Here's the drawing with two shaded views (mm, measured from the low corner). I have some questions. A direction names the side the tool comes from. Give positions to 0.01 mm unless a question says otherwise; leave off trailing zeros. Loops run counter-clockwise (first coordinate to the right, second up) from the corner with the lowest first, then second, coordinate; pieces in that order, holes last. Notation, with made-up numbers: (36, -30) -> (56, -30) arc R21 ccw to (56, -21) -> close; hole circle Ø5 at (49.5, -31.75). An arc over 180 degrees is marked (long way). Answer in a Markdown table with one row per item. Add a question column.
Item 1: If we section it at D-D (x = 2.5): Write out the boundary of the cut face in (y, z).
Item 2: If we section it at B-B (z = 6.25): Write out the boundary of the cut face in (x, y).
Item 3: If I drill on line 1 (X direction, y = 5.5, z = 6.25); line 2 (Y direction, x = 5.5, z = 1); line 3 (X direction, y = 6.5, z = 4.5), over which ranges is the centre line in solid material (lowest first)?
Item 4: For P1, Ø3, axis at x = 6.5, y = 5, coming from the +Z side; P2, Ø4, axis at y = 4.5, z = 8.5, coming from the -X side; P3, Ø6, axis at y = 6.5, z = 11, coming from the +X side, each with a flat end and sliding along its axis, tell me the tip position at first contact or that it passes through.
Item 5: We'd pull the mould along X, two halves only. Please class the marked faces 1, 2 and 3: released by +X, released by -X, zero draft, split by the parting line, or undercut.
Item 6: If we section it at A-A (x = 6.25): Write out the boundary of the cut face in (y, z).
Item 7: Which directions (+Z, -Z, +X, -X, +Y, -Y) give clear straight access to the entire face, cutting with the end or side of a thin tool? Please do the marked faces 4 and 5.
Item 8: If we section it at C-C (y = 4): Write out the boundary of the cut face in (x, z).
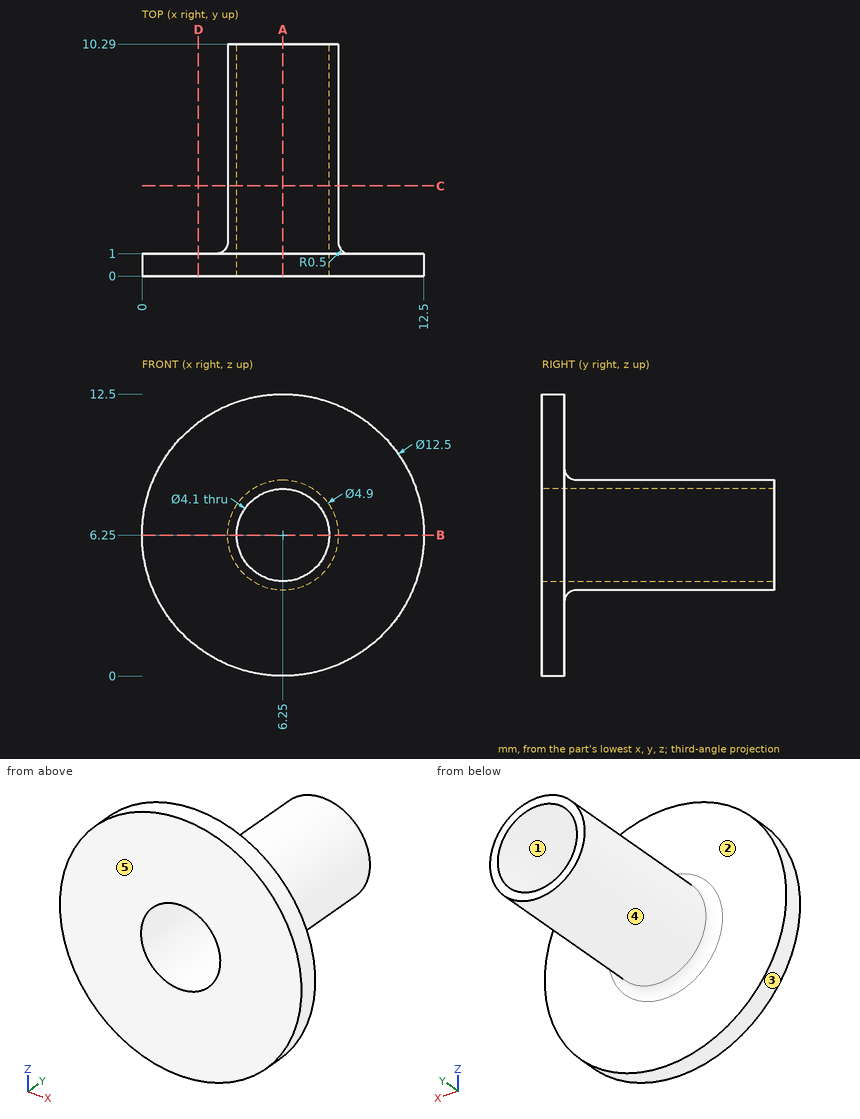
Recorded:
| question | item | result |
|---|---|---|
| 1 | outline | (0, 1.25) -> (1, 1.25) -> (1, 11.25) -> (0, 11.25) -> close |
| 2 | outline | (0, 0) -> (4.2, 0) -> (4.2, 10.29) -> (3.8, 10.29) -> (3.8, 1.5) arc R0.5 cw to (3.3, 1) -> (0, 1) -> close; (8.3, 0) -> (12.5, 0) -> (12.5, 1) -> (9.2, 1) arc R0.5 cw to (8.7, 1.5) -> (8.7, 10.29) -> (8.3, 10.29) -> close |
| 3 | line 1 | x = 3.8 to 4.2, 8.3 to 8.7 |
| 3 | line 2 | y = 0 to 1 |
| 3 | line 3 | x = 4.54 to 5.18, 7.32 to 7.96 |
| 4 | P1 | stops at z = 8.7 |
| 4 | P2 | stops at x = 3.81 |
| 4 | P3 | stops at x = 7.96 |
| 5 | face 1 | undercut |
| 5 | face 2 | zero draft |
| 5 | face 3 | split by the parting line |
| 6 | outline | (0, 0) -> (1, 0) -> (1, 3.3) arc R0.5 cw to (1.5, 3.8) -> (10.29, 3.8) -> (10.29, 4.2) -> (0, 4.2) -> close; (0, 8.3) -> (10.29, 8.3) -> (10.29, 8.7) -> (1.5, 8.7) arc R0.5 cw to (1, 9.2) -> (1, 12.5) -> (0, 12.5) -> close |
| 7 | face 4 | +Y |
| 7 | face 5 | +Z, -Z, +X, -X, -Y |
| 8 | outline | circle Ø4.9 at (6.25, 6.25); hole circle Ø4.1 at (6.25, 6.25) |
